Input: dimensioned drawing with shaded views. Units: mm. Origin: part minimum x, y, z. A direction names the side the tool comes from. Give positions to 0.01 mm unless a question says otherwise; leave off trailing zeros. Write each loop counter-clockwise with the first axis right and the second up, starting at its lowest first coordinate (ties: lowest second). Pieces come first, ordered by that corner, then holes.
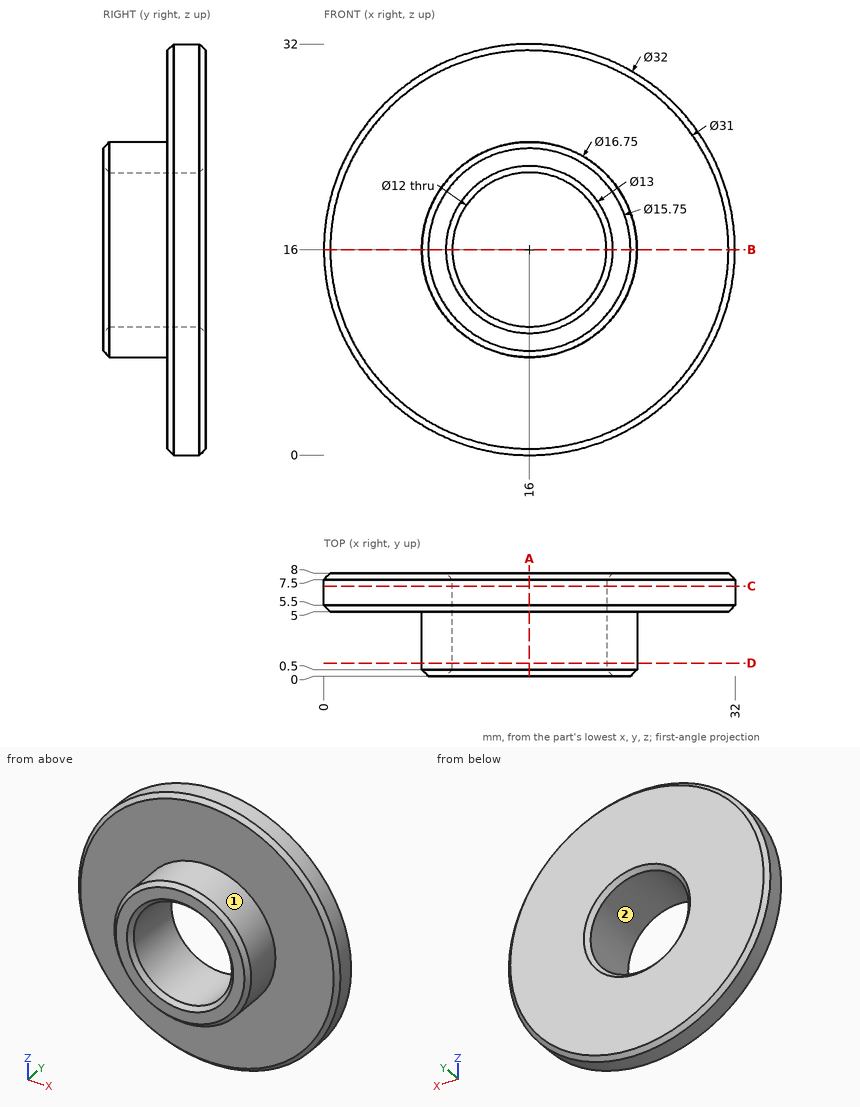
Item 1: Section B-B, the plane z = 16. Return the cut outline in (x, y) (3 decimals).
Found:
outline: (0, 5.5) - (0.5, 5) - (7.625, 5) - (7.625, 0.5) - (8.125, 0) - (9.5, 0) - (10, 0.5) - (10, 7.5) - (9.5, 8) - (0.5, 8) - (0, 7.5) - close; (22, 0.5) - (22.5, 0) - (23.875, 0) - (24.375, 0.5) - (24.375, 5) - (31.5, 5) - (32, 5.5) - (32, 7.5) - (31.5, 8) - (22.5, 8) - (22, 7.5) - close
Item 2: Line query: L1, parallel to Z at x = 16, y = 3.25 (3 decimals); L2, parallel to Y at x = 26, z = 13.5; L3, parallel to X at y = 3.5, z = 19. Output: solid intervals per line, ascending.
Found:
L1: z = 7.625 to 10, 22 to 24.375
L2: y = 5 to 8
L3: x = 8.18 to 10.8, 21.2 to 23.82
Item 3: Section C-C, the plane y = 7. Return the cut outline in (x, z), plus the area to 3 significant figures.
Found:
outline: circle Ø32 at (16, 16); hole circle Ø12 at (16, 16)
area: 691 mm2
Item 4: Pin query (flat end, axial travel): pin 1 Ø4 at (y, z) = (2, 26.5) entering from -X. Return the tip coordinate at first contact, or that it passes through.
Found:
pin 1: passes through
Item 5: Section A-A, the plane x = 16. Return the cut outline in (y, z) (3 decimals), plus the area to 3 significant figures.
Found:
outline: (0, 8.125) - (0.5, 7.625) - (5, 7.625) - (5, 0.5) - (5.5, 0) - (7.5, 0) - (8, 0.5) - (8, 9.5) - (7.5, 10) - (0.5, 10) - (0, 9.5) - close; (0, 22.5) - (0.5, 22) - (7.5, 22) - (8, 22.5) - (8, 31.5) - (7.5, 32) - (5.5, 32) - (5, 31.5) - (5, 24.375) - (0.5, 24.375) - (0, 23.875) - close
area: 82.5 mm2
Item 6: Section D-D, the plane y = 1. Return the cut outline in (x, z) (3 decimals), plus the area to 3 significant figures.
Found:
outline: circle Ø16.75 at (16, 16); hole circle Ø12 at (16, 16)
area: 107 mm2
Item 7: Reachability of the marked faces 1 and 2 from +Z, -Z, +X, -X, +Y, -Y: full face, straight path, thin tool, end or side. Return the list, or none.
Found:
face 1: -Y
face 2: +Y, -Y
